Solid Edge part; units mm, degrees
sketch "Sketch1" plane through (0, 0, 0) normal (0, 0, 1) x (1, 0, 0)
  line L0 (-70.5, -125) -> (70.5, -125)
  arc A0 (70.5, -125) -> (72.5, -123) centre (70.5, -123) ccw
  line L1 (72.5, -123) -> (72.5, 123)
  arc A1 (72.5, 123) -> (70.5, 125) centre (70.5, 123) ccw
  line L2 (70.5, 125) -> (-70.5, 125)
  arc A2 (-70.5, 125) -> (-72.5, 123) centre (-70.5, 123) ccw
  line L3 (-72.5, 123) -> (-72.5, -123)
  arc A3 (-70.5, -125) -> (-72.5, -123) centre (-70.5, -123) cw
extrude "Extrusionsausprägung_1" add sketch "Sketch1" along normal blind 2.5
hole "Bohrung_1" at (-44.9, -80, 0) direction (0, 0, 1) diameter 3.3 end up to next countersink diameter 6.3 countersink angle 120
hole "Hole1" at (44.9, -80, 0) direction (0, 0, 1) diameter 3.3 end up to next countersink diameter 6.3 countersink angle 120
hole "Hole2" at (-44.9, 80, 0) direction (0, 0, 1) diameter 3.3 end up to next countersink diameter 6.3 countersink angle 120
hole "Hole3" at (44.9, 80, 0) direction (0, 0, 1) diameter 3.3 end up to next countersink diameter 6.3 countersink angle 120
hole "Bohrung_5" at (-62.5, 112.5, 2.5) direction (0, 0, -1) diameter 6.4 end up to next
hole "Hole4" at (62.5, 112.5, 2.5) direction (0, 0, -1) diameter 6.4 end up to next
hole "Hole5" at (62.5, -112.5, 2.5) direction (0, 0, -1) diameter 6.4 end up to next
hole "Hole6" at (-62.5, -112.5, 2.5) direction (0, 0, -1) diameter 6.4 end up to next
properties material "Aluminium, 2024-T4"
Could you check a few things on this model? Use its own coordinates, in mm. Give positions to 0.01 mm unless a question says otherwise; leave off trailing zeros. Loops run counter-clockwise (first coordinate to the right, second up) from the corner with the lowest first, then second, coordinate; pieces in that order, holes last. Notation, with made-up numbers: (48, 78.25) -> (90, 78.25) arc R27 cw to (90, 107.25) -> close; hole circle Ø1 at (-13.75, 48). An arc over 180 degrees is marked (long way). Answer as CSV lines item,"result". Start each with the question number.
(1) If we section it at A-A on y = -112.5: Write out the boundary of the cut face in (x, z), then the cut area to 4 significant figures.
(2) I'm going to push flat-ended pins straight in: pin 1 Ø4.5 at (x, y) = (-44.9, -80) entering from -Z; pin 2 Ø5.5 at (x, y) = (44.9, -80) entering from -Z. Where does each tip first touch, or does it pass through?
(3) If we section it at B-B on x = -62.5: Write out the boundary of the cut face in (y, z).
(4) I need wall thicknesses on probe 1 along X at (y, z) = (-80, 1.9); probe 2 along X at (y, z) = (-112.5, 0.8); probe 3 along Y at (x, z) = (-62.5, 1.8). Which ranges of each line are inside material? Lowest first, please.
(5) We'd pull the mould along X, two halves only. Please class faces 1 (the cylindrical face through (-61.539, -115.552, 1.268)), 2 (the cylindrical face through (61.274, 109.544, 1.268)), 3 (the flat face through (-1, 2, 2.5)): released by +X, released by -X, zero draft, split by the parting line, or undercut.
Computed:
1,outline,"(-72.5, 0) -> (-65.7, 0) -> (-65.7, 2.5) -> (-72.5, 2.5) -> close; (-59.3, 0) -> (59.3, 0) -> (59.3, 2.5) -> (-59.3, 2.5) -> close; (65.7, 0) -> (72.5, 0) -> (72.5, 2.5) -> (65.7, 2.5) -> close"
1,area,"330.5 mm2"
2,pin 1,"stops at z = 0.52"
2,pin 2,"stops at z = 0.23"
3,outline,"(-125, 0) -> (-115.7, 0) -> (-115.7, 2.5) -> (-125, 2.5) -> close; (-109.3, 0) -> (109.3, 0) -> (109.3, 2.5) -> (-109.3, 2.5) -> close; (115.7, 0) -> (125, 0) -> (125, 2.5) -> (115.7, 2.5) -> close"
4,probe 1,"x = -72.5 to -46.55, -43.25 to 43.25, 46.55 to 72.5"
4,probe 2,"x = -72.5 to -65.7, -59.3 to 59.3, 65.7 to 72.5"
4,probe 3,"y = -125 to -115.7, -109.3 to 109.3, 115.7 to 125"
5,face 1,"undercut"
5,face 2,"undercut"
5,face 3,"zero draft"
